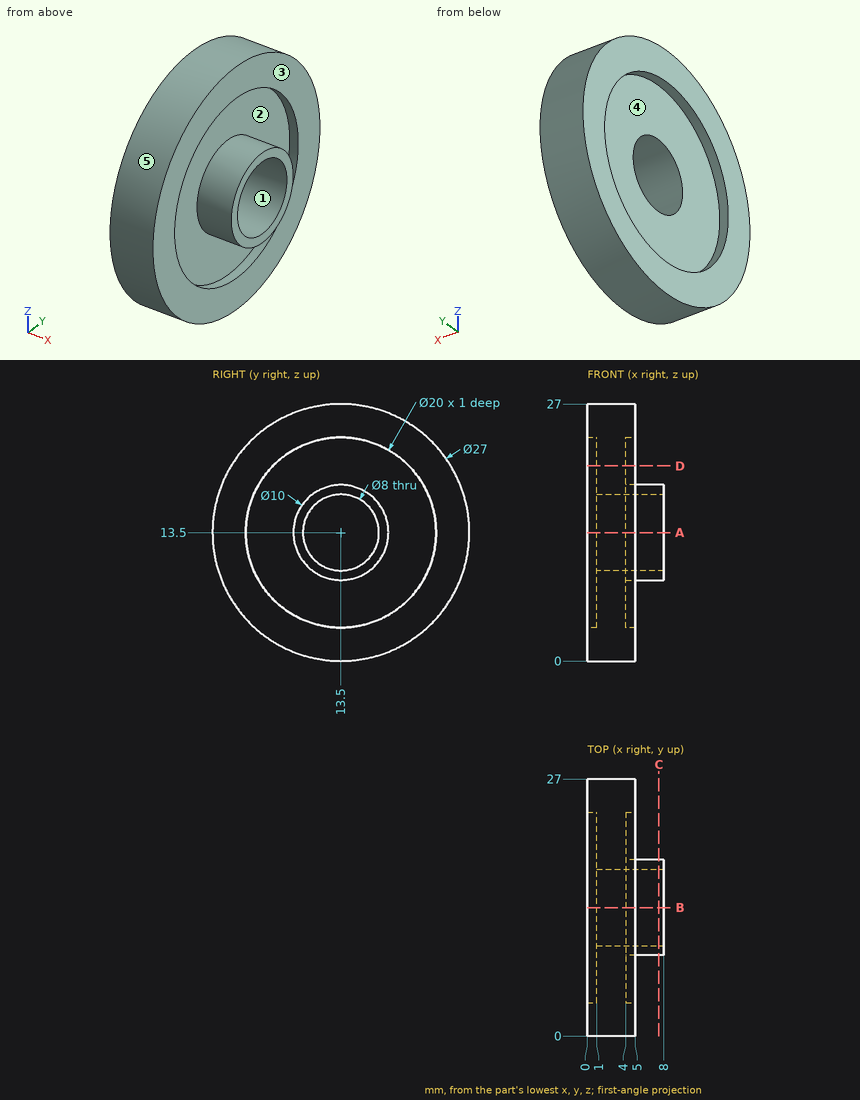
The figure shows three views and two pictorial views of one solid part (mm, origin at its lowest corner). Answer the questions. A direction names the side the tool comes from. Round coordinates to 2 decimals unless told otherwise and drop trailing zeros. Order: outer loops, then holes, each group sorted by start corner. A loop starts at its lowest first (then second) coordinate and runs counter-clockwise, first axis right, second up. Notation, with made-up numbers: M 77,62 L 124,62 A28 cw 124,80 Z; hole C 79.25,66 d8. An arc over 180 degrees is marked long. Answer in a Markdown table with one row per item. Add a question column.
1) Determine the mould class of the marked faces 3, 4 and 5 for opening direction Y: pulls with the +Y half, pulls with the -Y half, needs draft (parallel to the pull), parting line crosses it, or undercut.
2) Consider line 1 along Y through (x, z) = (4.25, 13.5); line 2 along Y through (x, z) = (0.6, 13.5); line 3 along Y through (x, z) = (6.25, 11). Determine where each line is inside the solid, lowest interval first. Write a range as from..to.
3) Which of the six approach directions +Z, -Z, +X, -X, +Y, -Y give full straight-line access (tool end or side, diameter ignored) to the marked faces 1 and 2?
4) The part is cut by section C-C on x = 7.5. Determine the outline of the cut face in (y, z), plus the area to 3 significant figures.
5) The part is cut by section D-D on z = 20.5. Determine the outline of the cut face in (x, y), plus the area to 3 significant figures.
6) Flat-ended cylindrical pins translate along their axes: pin 1 Ø2 at (x, y) = (5, 11.5) entering from -Z; pin 2 Ø3 at (x, z) = (1.5, 24.5) entering from -Y; pin 3 Ø1.5 at (y, z) = (15, 19) entering from -X. Find the tip coordinate at first contact, or state that the pin passes through.
7) The part is cut by section A-A on z = 13.5. Determine the outline of the cut face in (x, y).
Findings below:
| question | item | result |
|---|---|---|
| 1 | face 3 | needs draft |
| 1 | face 4 | undercut |
| 1 | face 5 | parting line crosses it |
| 2 | line 1 | y = 0..3.5, 8.5..9.5, 17.5..18.5, 23.5..27 |
| 2 | line 2 | y = 0..3.5, 23.5..27 |
| 2 | line 3 | y = 9.17..10.38, 16.62..17.83 |
| 3 | face 1 | +X, -X |
| 3 | face 2 | +X |
| 4 | outline | C 13.5,13.5 d10; hole C 13.5,13.5 d8 |
| 4 | area | 28.3 mm² |
| 5 | outline | M 0,1.96 L 5,1.96 L 5,6.36 L 4,6.36 L 4,20.64 L 5,20.64 L 5,25.04 L 0,25.04 L 0,20.64 L 1,20.64 L 1,6.36 L 0,6.36 Z |
| 5 | area | 86.9 mm² |
| 6 | pin 1 | stops at z = 0.04 |
| 6 | pin 2 | stops at y = 3.91 |
| 6 | pin 3 | stops at x = 1 |
| 7 | outline | M 0,0 L 5,0 L 5,3.5 L 4,3.5 L 4,8.5 L 8,8.5 L 8,9.5 L 1,9.5 L 1,3.5 L 0,3.5 Z; M 0,23.5 L 1,23.5 L 1,17.5 L 8,17.5 L 8,18.5 L 4,18.5 L 4,23.5 L 5,23.5 L 5,27 L 0,27 Z |
